The drawing under review shows one solid part. Ordinate dimensions are in mm from its lowest x, y, z. A direction names the side the tool comes from. Coordinates: 2 decimals unless noted, no trailing zeros. Order: outer loops, then holes, each group sorted by start corner. A loop starts at its lowest first (then second) coordinate and runs counter-clockwise, first axis right, second up.
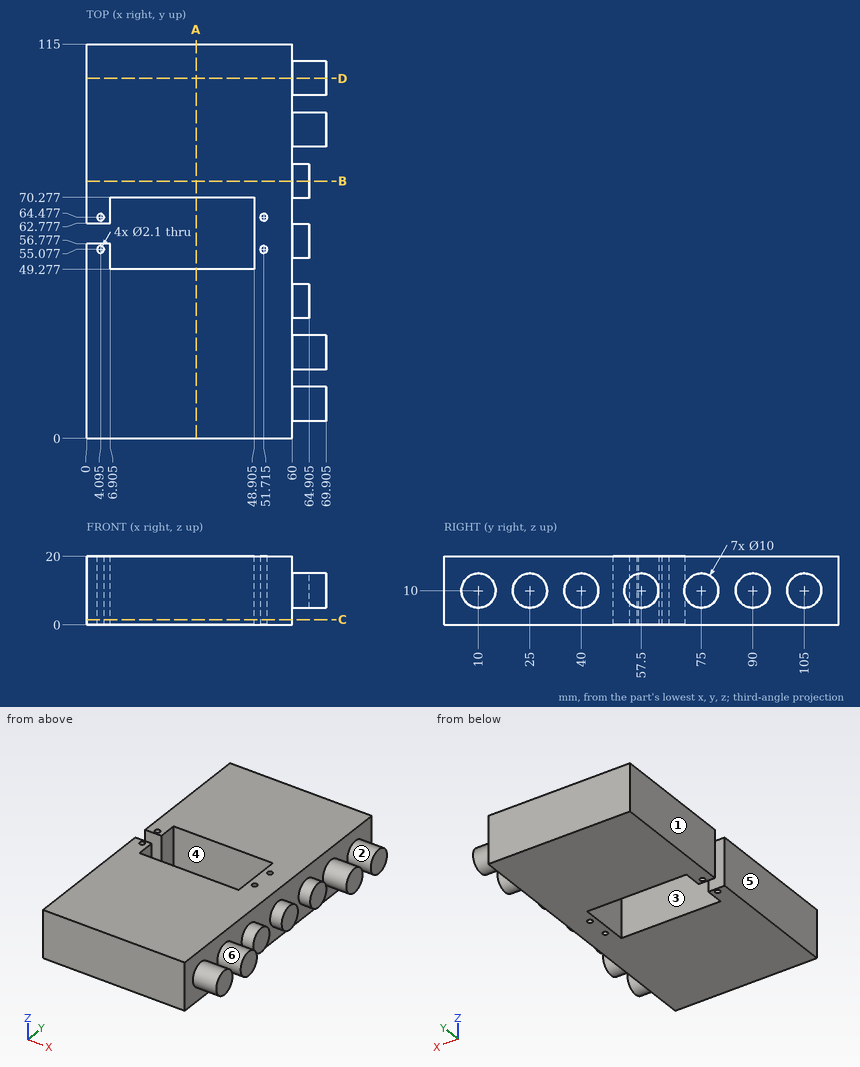
(1) Consider section C-C (z = 1.5). Give the number of separate pieces and of enclosed holes in the cut face, then the cut area to 3 significant figures.
(2) Consider section D-D (y = 105). Give the boundary of the cut face in (x, z) (1 decimal).
(3) Insertion check: pin 1 Ø1.9 at (x, y) = (4.09, 64.48) entering from -Z; pin 2 Ø2 at (y, z) = (68, 12.5) entering from +X; pin 3 Ø11 at (y, z) = (75.5, 8.5) entering from +X (1 decimal). Each pin has a flat end and moves straight along its axis. Give the tip position at first contact, or say it passes through.
(4) Tool access review of the marked faces 1, 2 and 3: name each direction out of +Z, -Z, +X, -X, +Y, -Y from which nothing blocks a thin tool from reaching the whole face with its end or side.
(5) Consider section B-B (y = 75). Give the boundary of the cut face in (x, z) (1 decimal), then the cut area to 3 significant figures.
(6) Consider section A-A (x = 32). Give the boundary of the cut face in (y, z).
(7) Wall thickness on line 1 (Y direction, x = 7, z = 4.75); line 2 (Y direction, x = 6, z = 3.5); line 3 (X direction, y = 47.5, z = 5): over which ranges is each line inside the solid? List them lowest first.
(8) The part is to be moulded in two halves that separate along X. For the marked faces 4, 5 and 6, say which applies: +X half, -X half, draft (parallel to the pull), parting line (faces both ways), or undercut.
Findings:
1. separate pieces: 1
1. enclosed holes: 4
1. area: 5,960 mm2
2. outline: (0, 0) - (60, 0) - (60, 5) - (69.9, 5) - (69.9, 15) - (60, 15) - (60, 20) - (0, 20) - close
3. pin 1: passes through
3. pin 2: stops at x = 60
3. pin 3: stops at x = 64.9
4. face 1: +Z, -Z, -X, +Y, -Y
4. face 2: +X
4. face 3: +Z, -Z
5. outline: (0, 0) - (60, 0) - (60, 5) - (64.9, 5) - (64.9, 15) - (60, 15) - (60, 20) - (0, 20) - close
5. area: 1,250 mm2
6. outline: (0, 0) - (49.28, 0) - (49.28, 20) - (0, 20) - close; (70.28, 0) - (115, 0) - (115, 20) - (70.28, 20) - close
7. line 1: y = 0 to 49.28, 70.28 to 115
7. line 2: y = 0 to 56.78, 62.78 to 115
7. line 3: x = 0 to 60
8. face 4: undercut
8. face 5: -X half
8. face 6: draft
